Part print with two shaded views. Sizes in mm from the minimum x, y, z corner. A direction names the side the tool comes from. Round coordinates to 2 decimals unless told otherwise and drop trailing zeros. Write each loop counter-clockwise with the first axis right and the second up, starting at its lowest first coordinate (ties: lowest second). Pieces come first, ordered by that corner, then holes. Notation, with made-up numbers: M 80.5,61.5 L 97.5,61.5 A18 ccw 97.5,75.5 Z; hole C 24.5,3 d8. An arc over 180 degrees is marked long. One line per question, with ' | ' between items. Start each with the question number.
1) Saw through at D-D (y = 12). List the corners of the cut face in (x, z), plus the area to 3 significant figures.
2) Saw through at C-C (z = 9). List the corners of the cut face in (x, y).
3) Tool access for the marked faces 4 and 5: list every direction of +Z, -Z, +X, -X, +Y, -Y with a clear straight run to the whole face (end or side of a thin tool).
4) Mould opens along Y. For the marked faces 1, 2 and 3 say: pulls with the +Y half, pulls with the -Y half, needs draft (parallel to the pull), parting line crosses it, or undercut.
5) Drop flat-ended pins along their axis: pin 1 Ø8.5 at (x, y) = (9, 9) entering from +Z; pin 2 Ø2 at (y, z) = (19.5, 9) entering from -X; pin 3 Ø9 at (y, z) = (6, 10) entering from -X; pin 4 Ø3 at (y, z) = (17, 6.5) entering from -X. Give the stop position or say it passes through.
6) Wall check: probe 1 along Y at (x, z) = (8, 0.8); probe 2 along Y at (x, z) = (22.25, 9); probe 3 along X at (y, z) = (19.5, 0.5). Give the ranges that are in metal, low to high. Write a range as [from, to].
7) Saw through at A-A (x = 8). List the corners of the cut face in (y, z).
8) Saw through at B-B (y = 5). List the corners of the cut face in (x, z), plus the area to 3 significant figures.
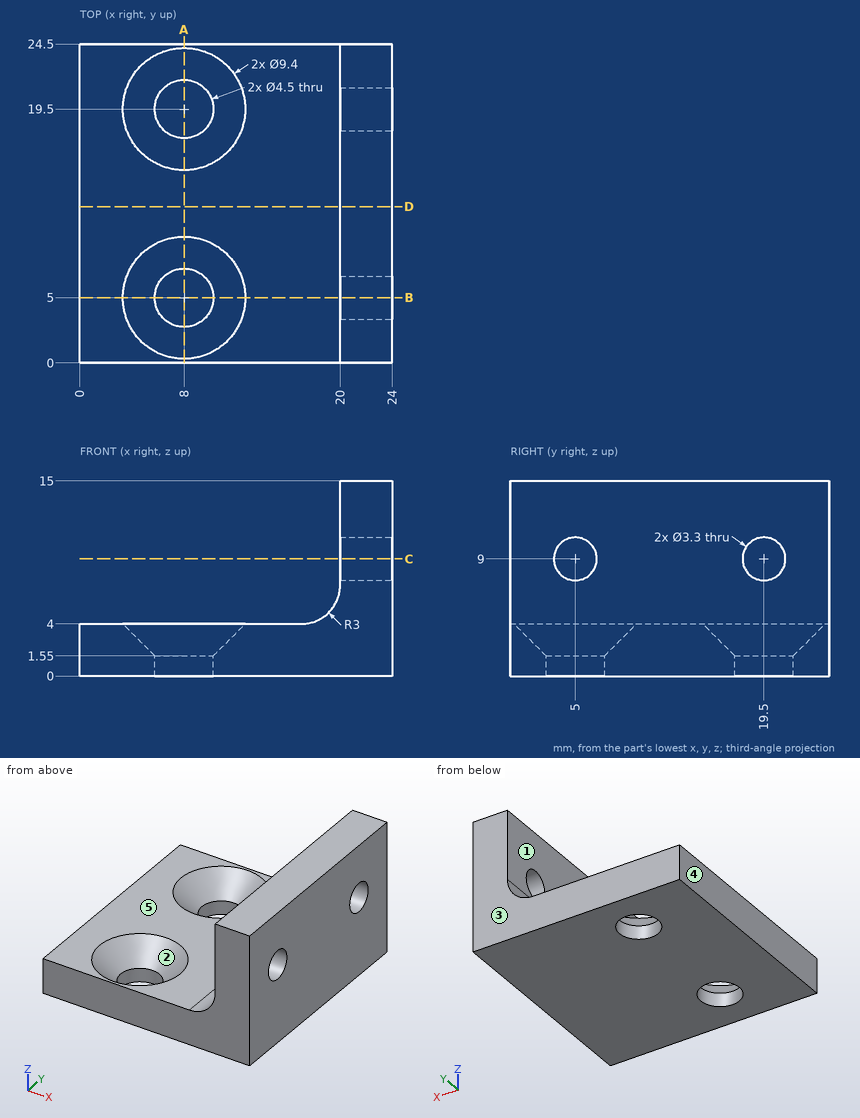
Answer key:
1) outline: M 0,0 L 24,0 L 24,15 L 20,15 L 20,7 A3 cw 17,4 L 0,4 Z | area: 142 mm2
2) outline: M 20,0 L 24,0 L 24,3.35 L 20,3.35 Z; M 20,6.65 L 24,6.65 L 24,17.85 L 20,17.85 Z; M 20,21.15 L 24,21.15 L 24,24.5 L 20,24.5 Z
3) face 4: +Z, -Z, -X, +Y, -Y | face 5: +Z, -X, +Y, -Y
4) face 1: needs draft | face 2: undercut | face 3: pulls with the +Y half
5) pin 1: stops at z = 4 | pin 2: passes through | pin 3: stops at x = 19.6 | pin 4: stops at x = 19.24
6) probe 1: y = [0, 2.75], [7.25, 17.25], [21.75, 24.5] | probe 2: y = [0, 3.35], [6.65, 17.85], [21.15, 24.5] | probe 3: x = [0, 5.75], [10.25, 24]
7) outline: M 0,0 L 2.75,0 L 2.75,1.55 L 0.3,4 L 0,4 Z; M 7.25,0 L 17.25,0 L 17.25,1.55 L 14.8,4 L 9.7,4 L 7.25,1.55 Z; M 21.75,0 L 24.5,0 L 24.5,4 L 24.2,4 L 21.75,1.55 Z
8) outline: M 0,0 L 5.75,0 L 5.75,1.55 L 3.3,4 L 0,4 Z; M 10.25,0 L 24,0 L 24,7.35 L 20,7.35 L 20,7 A3 cw 17,4 L 12.7,4 L 10.25,1.55 Z; M 20,10.65 L 24,10.65 L 24,15 L 20,15 Z | area: 105 mm2
